Design review of the part shown in the three views and the two pictorial views. Dimensions are in mm from the part's minimum x, y and z. A direction names the side the tool comes from. Give positions to 0.01 mm unless a question says otherwise; leave off trailing zeros. Write each loop counter-clockwise with the first axis right and the second up, starting at its lowest first coordinate (ties: lowest second). Pieces come first, ordered by that corner, then holes. Notation, with made-up numbers: (-11.5, -16.75) -> (4.5, -16.75) arc R21 cw to (4.5, 20.25) -> close; hole circle Ø10 at (66.25, -0.5). An arc over 180 degrees is marked (long way). Return JSON: item names as keys, results as strings. Group by question number.
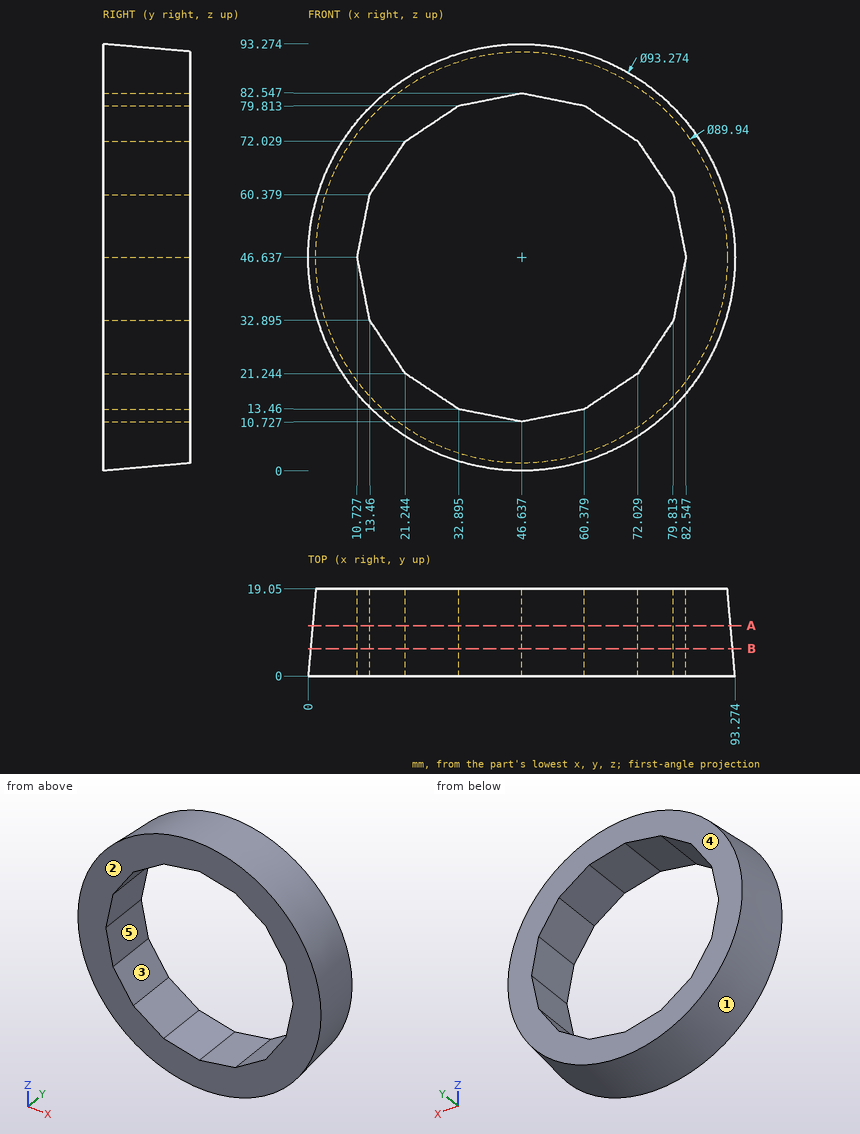
Q1. Tool access review of the marked faces 4 and 5: name each direction out of +Z, -Z, +X, -X, +Y, -Y from which nothing blocks a thin tool from reaching the whole face with its end or side.
Q2. Mouldability with a two-part tool opening along Z and no side actions: class the marked faces 1, 2 and 3 as +Z half, -Z half, draft (parallel to the pull), parting line (faces both ways), or undercut.
Q3. Take a section at A-A, the plane y = 11. Give the boundary of the cut face in (x, z) (1 decimal), plus the area to 3 significant figures.
Q4. Insertion check: pin 1 (4 mm diameter, centred on y = 4, z = 33, fed in from +X); pin 2 (5 mm diameter, centred on x = 74.5, y = 3.5, fed in from -Z) (1 decimal); pin 3 (2 mm diameter, centred on x = 71.5, y = 11.5, fed in from +Z). Each pin has a flat end and moves straight along its axis. Give the tip position at first contact, or say it passes through.
Q5. For L1, parallel to Z at x = 77.5, y = 15 (1 decimal); L2, parallel to Z at x = 43, y = 16.75; L3, parallel to X at y = 3, z = 51.5 (1 decimal), list the stretches that pass through material, from the lowest coordinate up. Write a range as from..to.
Q6. Take a section at B-B, the plane y = 6. Give the boundary of the cut face in (x, z) (1 decimal), plus the area to 3 significant figures.
Final values:
{
 "1": {"face 4": "+Z, -Z, +X, -X, +Y", "face 5": "+Y, -Y"},
 "2": {"face 1": "parting line", "face 2": "draft", "face 3": "undercut"},
 "3": {"outline": "circle Ø91.3 at (46.6, 46.6); hole (10.7, 46.6) -> (13.5, 32.9) -> (21.2, 21.2) -> (32.9, 13.5) -> (46.6, 10.7) -> (60.4, 13.5) -> (72, 21.2) -> (79.8, 32.9) -> (82.5, 46.6) -> (79.8, 60.4) -> (72, 72) -> (60.4, 79.8) -> (46.6, 82.5) -> (32.9, 79.8) -> (21.2, 72) -> (13.5, 60.4) -> close", "area": "2,610 mm²"},
 "4": {"pin 1": "stops at x = 91.47", "pin 2": "stops at z = 7.8", "pin 3": "stops at z = 85.54"},
 "5": {"L1": "z = 13.4..29.4, 63.8..79.8", "L2": "z = 1.61..11.45, 81.82..91.66", "L3": "x = 0.5..11.7, 81.6..92.8"},
 "6": {"outline": "circle Ø92.2 at (46.6, 46.6); hole (10.7, 46.6) -> (13.5, 32.9) -> (21.2, 21.2) -> (32.9, 13.5) -> (46.6, 10.7) -> (60.4, 13.5) -> (72, 21.2) -> (79.8, 32.9) -> (82.5, 46.6) -> (79.8, 60.4) -> (72, 72) -> (60.4, 79.8) -> (46.6, 82.5) -> (32.9, 79.8) -> (21.2, 72) -> (13.5, 60.4) -> close", "area": "2,730 mm²"}
}
